For this review, take the finished solid that the model builds, in its own axes (mm). Face numbers are marked on the shaded views. A direction names the side the tool comes from. Give positions to 0.01 mm unless a question says otherwise; leave off trailing zeros. Order: outer loops, then holes, each group sorted by start corner. A loop starts at its lowest first (then second) coordinate and runs counter-clockwise, first axis right, second up. Notation, with made-up numbers: (70.25, 26.5) - (112.25, 26.5) arc R13 cw to (112.25, 34.5) - close; hole circle Ø8 at (32.25, 30). An arc over 180 degrees is marked (long way). Use a Markdown table: item, result. Add a question column.
1) We need section A-A on y = 11. Write out the cut boundary in (x, z), then the cut area to 3 significant figures.
2) Machinability: for the marked faces 1, 2 and 3, which of the approach directions +Z, -Z, +X, -X, +Y, -Y give a long, thin tool a straight path to every point of the face, cutting with its end or side? Answer none if there is none.
3) Wall thickness on L1, parallel to Y at x = -38.5, z = 19.75; L2, parallel to X at y = 32.5, z = 10.5; L3, parallel to Z at x = -24, y = 32.5: over which ranges is each line inside the solid? List them lowest first.
4) Mouldability with a two-part tool opening along X and no side actions: class the marked faces 4, 5 and 6 as released by +X, released by -X, zero draft, split by the parting line, or undercut.
5) We need section B-B on x = -25. Write out the cut boundary in (y, z), then the cut area to 3 significant figures.
6) Clearance check with flat-ended pins moving along their axes: P1, Ø2, axis at x = -10.5, z = 24.5, coming from the +Y side; P2, Ø3, axis at y = -17, z = 23.5, coming from the +X side (3 decimals); P3, Ø8, axis at x = -23.5, y = -24, coming from the +Z side. State where each tip first meets the part, or that it passes through.
```python
from build123d import *

# Parameters (mm, degrees)
F0_W     = 74.4920149446
F0_H     = 77.3611664772
F1_DEPTH = 25
F2_R     = 5
F3_T     = -2.5
F5_D     = 5
F5_DEPTH = 12
F5_TIP   = 1.5021515476


# Not quite as in the source:
# - a shell that OpenCascade refuses in one call is made with other operations: the cavity is built on its own and cut out


with BuildPart() as f1:
    # F0 (on Top) → F1 (new body)
    with BuildSketch(Plane.XY):
        with Locations((-7.9336054623, -1.4722160995)):
            Rectangle(F0_W, F0_H)
    extrude(amount=F1_DEPTH)

    # F2
    f2_edges = [f1.edges().sort_by_distance(p)[0] for p in [
        (29.312402, -40.152799, 12.5),
        (29.312402, -1.472216, 25),
        (-7.933605, -40.152799, 25),
        (-45.179613, -1.472216, 25),
        (-7.933605, 37.208367, 25),
        (29.312402, -1.472216, 0),
        (-7.933605, -40.152799, 0),
        (29.312402, 37.208367, 12.5),
        (-45.179613, -40.152799, 12.5),
        (-45.179613, 37.208367, 12.5),
        (-45.179613, -1.472216, 0),
        (-7.933605, 37.208367, 0),
    ]]
    fillet(f2_edges, radius=F2_R)

    # F3: a shell. OpenCascade refuses it in one call, so the cavity is built on its own and cut out:
    # the body offset inwards by the wall thickness, plus a prism from it out through each open face.
    f3_core = offset(f1.part, amount=F3_T, mode=Mode.PRIVATE)
    f3_exits = [f3_core.faces().sort_by_distance(p)[0] for p in [
        (-7.933605, -1.472216, 22.5),
    ]]
    add(f3_core, mode=Mode.SUBTRACT)
    extrude(f3_exits, amount=-F3_T, mode=Mode.SUBTRACT)

    # F5
    with Locations(Plane.YZ.offset(29.31240201)):
        with Locations((-21.4438159019, 12.2315008193)):
            Hole(F5_D / 2, depth=F5_DEPTH)
            with Locations((0, 0, -(F5_DEPTH + F5_TIP / 2))):  # 118° drill point
                Cone(0, F5_D / 2, F5_TIP, mode=Mode.SUBTRACT)


solid = f1.part
```
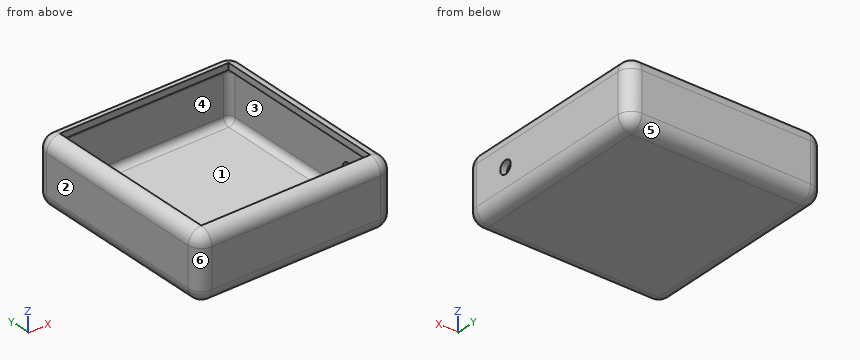
Checked values:
| question | item | result |
|---|---|---|
| 1 | outline | (-45.18, 5) arc R5 ccw to (-40.18, 0) - (24.31, 0) arc R5 ccw to (29.31, 5) - (29.31, 20) arc R5 ccw to (24.31, 25) - (24.31, 22.5) arc R2.5 cw to (26.81, 20) - (26.81, 5) arc R2.5 cw to (24.31, 2.5) - (-40.18, 2.5) arc R2.5 cw to (-42.68, 5) - (-42.68, 20) arc R2.5 cw to (-40.18, 22.5) - (-40.18, 25) arc R5 ccw to (-45.18, 20) - close |
| 1 | area | 295 mm² |
| 2 | face 1 | +Z |
| 2 | face 2 | +Z, -Z, -X, +Y, -Y |
| 2 | face 3 | none |
| 3 | L1 | -40.15 to -37.65, 34.71 to 37.21 |
| 3 | L2 | -45.17 to -42.66, 26.8 to 29.3 |
| 3 | L3 | 0.01 to 2.52, 22.48 to 24.99 |
| 4 | face 4 | undercut |
| 4 | face 5 | zero draft |
| 4 | face 6 | released by -X |
| 5 | outline | (-40.15, 5) arc R5 ccw to (-35.15, 0) - (32.21, 0) arc R5 ccw to (37.21, 5) - (37.21, 20) arc R5 ccw to (32.21, 25) - (32.21, 22.5) arc R2.5 cw to (34.71, 20) - (34.71, 5) arc R2.5 cw to (32.21, 2.5) - (-35.15, 2.5) arc R2.5 cw to (-37.65, 5) - (-37.65, 20) arc R2.5 cw to (-35.15, 22.5) - (-35.15, 25) arc R5 ccw to (-40.15, 20) - close |
| 5 | area | 302 mm² |
| 6 | P1 | y = 35.78 |
| 6 | P2 | x = 28.895 |
| 6 | P3 | z = 2.5 |
